from build123d import *

# Parameters (mm, degrees)
F1_DEPTH  = 25
F2_SIZE   = 20
F3_T      = -5
F4_R      = 6.985
F5_DEPTH  = 25
F6_R      = 7.5
F7_DEPTH  = 25
F8_R      = 6
F10_DEPTH = 21
F11_R     = 3.175
F12_DEPTH = 25


with BuildPart() as f1:
    # F0 (on Front) → F1 (new body)
    with BuildSketch(Plane.XZ):
        with BuildLine():
            ThreePointArc((33.383667, 12.5), (24.59687, 33.713203), (3.383667, 42.5))
            Line((3.383667, 42.5), (-3.383667, 42.5))
            ThreePointArc((-3.383667, 42.5), (-24.59687, 33.713203), (-33.383667, 12.5))
            Line((-33.383667, 12.5), (-33.383667, -42.5))
            Line((-33.383667, -42.5), (33.383667, -42.5))
            Line((33.383667, -42.5), (33.383667, 12.5))
        make_face()
    extrude(amount=F1_DEPTH)

    # F2
    f2_edges = [f1.edges().sort_by_distance(p)[0] for p in [
        (-33.383667, -25, -15),
    ]]
    chamfer(f2_edges, length=F2_SIZE)

    # F3
    f3_openings = [f1.faces().sort_by_distance(p)[0] for p in [
        (0, 0, -2.614615),
    ]]
    offset(amount=F3_T, openings=f3_openings)

    # F4 (on face) → F5 (cut)
    with BuildSketch(Plane(origin=(0, 0, -42.5), x_dir=(1, 0, 0), z_dir=(0, 0, -1))):
        with Locations((0, 9.917389)):
            Circle(F4_R)
    extrude(amount=-F5_DEPTH, mode=Mode.SUBTRACT)

    # F6 (on face) → F7 (join, through all)
    with BuildSketch(Plane.XZ.offset(25)):
        with Locations((0, 14.338327)):
            Circle(F6_R)
    extrude(amount=-F7_DEPTH)

    # F8 (on face) → F10 (cut, through all)
    with BuildSketch(Plane.XZ.offset(25)):
        with Locations((0, 14.338327)):
            Circle(F8_R)
    extrude(amount=-F10_DEPTH, mode=Mode.SUBTRACT)

    # F11 (on face) → F12 (cut, through all)
    with BuildSketch(Plane.XZ.offset(25)):
        with Locations((0, 14.338327)):
            Circle(F11_R)
    extrude(amount=-F12_DEPTH, mode=Mode.SUBTRACT)


solid = f1.part
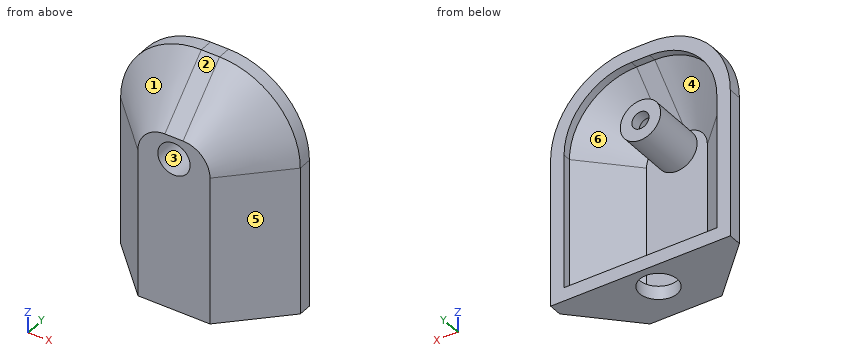
CAD build for the part. Positions are in the model's coordinates, mm. Face numbers are marked on the shaded views. A direction names the side the tool comes from. Round coordinates to 2 decimals unless told otherwise and drop trailing zeros. Write each loop counter-clockwise with the first axis right and the second up, starting at its lowest first coordinate (ties: lowest second). Pieces come first, ordered by that corner, then holes. Notation, with made-up numbers: (22.5, -6) -> (76.5, -6) arc R22 ccw to (76.5, 21) -> close; hole circle Ø10 at (52, 24). An arc over 180 degrees is marked (long way). Answer as a JSON object with one key per item and string values.
(1) Band-saw the part on A-A, the plane y = -2. List the corners of the cut face in (x, z) (3 decimals).
Reported:
{"outline": "(-33.384, -42.5) -> (33.384, -42.5) -> (33.384, 12.5) arc R30 ccw to (3.384, 42.5) -> (-3.384, 42.5) arc R30 ccw to (-33.384, 12.5) -> close; circle Ø15 at (0, 14.338); hole (-28.384, -37.5) -> (28.384, -37.5) -> (28.384, 12.5) arc R25 ccw to (3.384, 37.5) -> (-3.384, 37.5) arc R25 ccw to (-28.384, 12.5) -> close; hole circle Ø6.35 at (0, 14.338)"}
(2) Band-saw the part on B-B, the plane y = -9. List the corners of the cut face in (x, z).
Reported:
{"outline": "(-29.38, -42.5) -> (-6.92, -42.5) -> (-6.92, -37.5) -> (-22.31, -37.5) -> (-22.31, 12.5) arc R18.93 cw to (-3.38, 31.43) -> (3.38, 31.43) arc R18.93 cw to (22.31, 12.5) -> (22.31, -37.5) -> (6.92, -37.5) -> (6.92, -42.5) -> (29.38, -42.5) -> (29.38, 12.5) arc R26 ccw to (3.38, 38.5) -> (-3.38, 38.5) arc R26 ccw to (-29.38, 12.5) -> close; circle Ø15 at (0, 14.34); hole circle Ø12 at (0, 14.34)"}
(3) Two-plate mould, pull along X, no slides. Class the marked faces 1, 2, 3 and 4: +X half, -X half, draft (parallel to the pull), parting line (faces both ways), or undercut.
Reported:
{"face 1": "-X half", "face 2": "draft", "face 3": "undercut", "face 4": "undercut"}
(4) Which spindle directions (+Z, -Z, +X, -X, +Y, -Y) get a long thin tool onto all of the face, cutting with end or side? Do the marked faces 5 and 6. Say none if no direction does.
Reported:
{"face 5": "+Z, -Z, +X, -Y", "face 6": "+Y"}
(5) Band-saw the part on D-D, the plane z = -25. List the corners of the cut face in (x, y), then the cut area to 3 significant figures.
Reported:
{"outline": "(-33.38, -5) -> (-13.38, -25) -> (13.38, -25) -> (33.38, -5) -> (33.38, 0) -> (28.38, 0) -> (28.38, -2.93) -> (11.31, -20) -> (-11.31, -20) -> (-28.38, -2.93) -> (-28.38, 0) -> (-33.38, 0) -> close", "area": "425 mm^2"}
(6) Pin check, flat tips, straight feed: P1, Ø10, axis at x = 6, y = -13.5, coming from the +Z side; P2, Ø1.5, axis at x = -15, z = 23.5, coming from the -Y side; P3, Ø4, axis at y = -14, z = -26.5, coming from the +X side. Stop position of each tip, or through.
Reported:
{"P1": "stops at z = 38.89", "P2": "stops at y = -19.75", "P3": "stops at x = 26.38"}
(7) Probe probe 1 along Z at (x, y) = (0, -2.3); probe 2 along X at (y, z) = (-2.5, -19.5); probe 3 along X at (y, z) = (-2.75, 15). List the from-to ranges inside material, lowest first. Write a range as [from, to].
Reported:
{"probe 1": "z = [-42.5, -37.5], [6.84, 11.16], [17.51, 21.84], [37.5, 42.5]", "probe 2": "x = [-33.38, -28.38], [28.38, 33.38]", "probe 3": "x = [-33.28, -28.26], [-7.47, -3.11], [3.11, 7.47], [28.26, 33.28]"}
(8) Band-saw the part on C-C, the plane x = 0. List the corners of the cut face in (y, z), then the cut area to 3 significant figures.
Reported:
{"outline": "(-25, -42.5) -> (-16.9, -42.5) -> (-16.9, -37.5) -> (-20, -37.5) -> (-20, 6.84) -> (0, 6.84) -> (0, 11.16) -> (-4, 11.16) -> (-4, 8.34) -> (-25, 8.34) -> close; (-25, 20.34) -> (-4, 20.34) -> (-4, 17.51) -> (0, 17.51) -> (0, 21.84) -> (-18.59, 21.84) -> (-2.93, 37.5) -> (0, 37.5) -> (0, 42.5) -> (-5, 42.5) -> (-25, 22.5) -> close; (-2.93, -42.5) -> (0, -42.5) -> (0, -37.5) -> (-2.93, -37.5) -> close", "area": "522 mm^2"}
